Geometry: final body of the model. Coordinates: model frame, mm. A direction names the side the tool comes from. Give positions to 0.01 mm unless a question says otherwise; leave off trailing zeros. Loops run counter-clockwise (first coordinate to the right, second up) from the corner with the lowest first, then second, coordinate; pieces in that order, holes last. Notation, with made-up numbers: (50.25, -8.75) -> (92.25, -8.75) arc R16 cw to (92.25, -2.75) -> close; hole circle Ø11 at (39.25, 17.5). An arc over 180 degrees is marked (long way). Answer in a Markdown table with one row per item. Add a question column.
1) Section query B-B (y = -1.25). Return the cut outline in (x, z).
2) First-contact query: P1, Ø23.5, axis at x = 0, z = 0, coming from the +Y side; P2, Ø4, axis at y = 2.5, z = -5.5, coming from the -X side. Flat tips, straight axial feed; report the tip coordinate or a pass-through.
3) Draft query along Z for faces 3 (the flat face through (1, -3, 10)), 4 (the cylindrical face through (11.848, 2.465, -1.556)), 5 (the flat face through (0, -2.6, 2)), 6 (the cylindrical face through (2.703, 2.465, 8.584)). Return one class per face: +Z half, -Z half, draft (parallel to the pull), parting line (faces both ways), or undercut.
4) Section query A-A (y = 3.5). Return the cut outline in (x, z), plus the area to 3 significant figures.
5) Access query for faces 1 (the flat face through (9, 5, 2)), 2 (the flat face through (0, 0, 0)). Directions: +Z, -Z, +X, -X, +Y, -Y. A direction counts if a zero-diameter tool reaches every point of the face in a straight line with its end or side. Return the directions, or none.
6) Line query: line 1 (X direction, y = 2.5, z = 0); line 2 (Y direction, x = 11, z = 16.5); line 3 (Y direction, x = -6, z = 38). Output: solid intervals per line, ascending. Write a range as from..to.
```python
from build123d import *

# Parameters (mm, degrees)
SKETCH_1_R          = 11.95
SKETCH_1_R_2        = 9
EXTRUDE_1_DEPTH     = 5
SKETCH_2_R          = 44
EXTRUDE_2_DEPTH     = 3
FILLET_1_R          = 3
CUT_EXTRUDE_1_DEPTH = 0.4


with BuildPart() as part:
    # Эскиз1 → Бобышка-Вытянуть1 (new body)
    with BuildSketch(Plane(origin=(0, 0, 0), x_dir=(1, 0, 0), z_dir=(0, 1, 0))):
        with Locations(Location((0, 0, 0), (0, 0, 270))):
            Circle(SKETCH_1_R)
        with Locations(Location((0, 0, 0), (0, 0, 270))):
            Circle(SKETCH_1_R_2, mode=Mode.SUBTRACT)
    extrude(amount=EXTRUDE_1_DEPTH)

    # Эскиз2 → Бобышка-Вытянуть2 (add)
    with BuildSketch(Plane.XZ):
        with Locations(Location((0, 0, 0), (0, 0, 270))):
            Circle(SKETCH_2_R)
    extrude(amount=EXTRUDE_2_DEPTH)

    # Скругление1
    fillet_1_edges = [part.edges().sort_by_distance(p)[0] for p in [
        (0, -3, 44),
    ]]
    fillet(fillet_1_edges, radius=FILLET_1_R - 0.0001)  # a hair under: the kernel refuses the full size

    # Эскиз3 → Вырез-Вытянуть1 (cut)
    with BuildSketch(Plane.XZ.offset(3)):
        with BuildLine():
            Line((9.954559223, -5.855217729), (17.0939823, -6.624448498))
            add(Edge.make_bspline(
                [(17.0939823, -6.624448498), (16.954374573, -7.060364037), (16.67246957, -7.940593052), (16.082570182, -9.220685029), (15.367854468, -10.479237732), (14.549468275, -11.738227045), (13.598128393, -12.976714181), (12.508174471, -14.188327514), (11.307260102, -15.391109491), (9.994571436, -16.559013497), (8.599176625, -17.665541174), (7.097641414, -18.617186253), (5.53477836, -19.420340753), (3.908983058, -20.092788159), (2.213013482, -20.604345047), (0.449135236, -20.981542054), (-1.382110347, -21.198678471), (-2.625007466, -21.22599593), (-3.254575393, -21.239833113)],
                knots=[0, 0, 0, 0, 0.821440156, 1.658705401, 2.525323128, 3.419405186, 4.353419828, 5.32681938, 6.344399772, 7.404443113, 8.481060479, 9.538977106, 10.591299887, 11.633537695, 12.694215778, 13.768160887, 14.869500701, 16, 16, 16, 16], degree=3))
            add(Edge.make_bspline(
                [(-3.254575393, -21.239833113), (-4.037474252, -21.210468003), (-5.585963904, -21.152386976), (-7.859698842, -20.739484748), (-10.031214503, -20.033002378), (-12.082905697, -19.06267493), (-13.983263507, -17.838479622), (-15.628310659, -16.302835445), (-17.068788245, -14.551786811), (-18.226388665, -12.538555624), (-19.140015512, -10.335429034), (-19.780294703, -7.963227163), (-20.191471581, -5.448805692), (-20.238000287, -3.721455618), (-20.261786931, -2.838390806)],
                knots=[0, 0, 0, 0, 0.998551589, 1.975027533, 2.936744805, 3.903838964, 4.863557655, 5.807675034, 6.763178998, 7.745855275, 8.758641806, 9.797744155, 10.874151411, 12, 12, 12, 12], degree=3))
            add(Edge.make_bspline(
                [(-20.261786931, -2.838390806), (-20.253583862, -2.249072754), (-20.237148757, -1.068355571), (-20.071493014, 0.692734171), (-19.824593654, 2.443807008), (-19.457520681, 4.175543157), (-19.00443369, 5.89924412), (-18.436371871, 7.60283942), (-17.771918435, 9.296625216), (-17.009212067, 10.961487215), (-16.169576767, 12.570831605), (-15.246119859, 14.076076683), (-14.290825473, 15.491991281), (-13.257769645, 16.789715189), (-12.155533796, 17.973523587), (-11.00356969, 19.054320976), (-9.797035153, 20.040082521), (-8.518689542, 20.899962793), (-7.204489818, 21.664382583), (-5.862524589, 22.334760878), (-4.485868659, 22.886891815), (-3.083314583, 23.339978114), (-1.660006861, 23.708336607), (-0.208394214, 23.955377865), (1.268817222, 24.120842874), (2.265803014, 24.136773037), (2.767059223, 24.144782271)],
                knots=[0, 0, 0, 0, 1.075906032, 2.155611451, 3.227554832, 4.30373447, 5.38628686, 6.480642286, 7.581143633, 8.707391042, 9.82337293, 10.893692135, 11.930684225, 12.940768785, 13.919223559, 14.881988069, 15.823529777, 16.761054785, 17.692163021, 18.598508727, 19.497917784, 20.397951545, 21.288749041, 22.180057169, 23.084984307, 24, 24, 24, 24], degree=3))
            add(Edge.make_bspline(
                [(2.767059223, 24.144782271), (3.396819449, 24.13271298), (4.624674455, 24.109181262), (6.419415658, 23.873617188), (8.114533072, 23.493780483), (9.71479097, 22.957293415), (11.228369978, 22.293366902), (12.626669407, 21.438368521), (13.932702912, 20.448929523), (15.134462193, 19.318054618), (16.221199996, 18.057248477), (17.152473609, 16.665333162), (17.973572218, 15.181251724), (18.615932964, 13.571276078), (19.12246379, 11.857059969), (19.479861685, 10.030309351), (19.69885311, 8.096457894), (19.72490677, 6.769573083), (19.738213069, 6.091897656)],
                knots=[0, 0, 0, 0, 1.079196217, 2.10412856, 3.097265039, 4.052997914, 4.993829394, 5.924450447, 6.855882321, 7.798592485, 8.748507102, 9.702980304, 10.665060364, 11.651045023, 12.668191174, 13.725659051, 14.838433479, 16, 16, 16, 16], degree=3))
            add(Edge.make_bspline(
                [(19.738213069, 6.091897656), (19.711530906, 5.012347464), (19.657182115, 2.813415932), (19.336536232, 0.637210246), (19.173309223, -0.470602344)],
                knots=[0, 0, 0, 0, 0.981886135, 2, 2, 2, 2], degree=3))
            Line((19.173309223, -0.470602344), (-12.569479239, -0.470602344))
            add(Edge.make_bspline(
                [(-12.569479239, -0.470602344), (-12.686010265, -0.684825825), (-12.905708031, -1.088704703), (-13.155238164, -1.702843602), (-13.305966259, -2.286193686), (-13.328203982, -2.669377879), (-13.338710008, -2.850410037)],
                knots=[0, 0, 0, 0, 1.156942796, 2.181202349, 3.140724307, 4, 4, 4, 4], degree=3))
            add(Edge.make_bspline(
                [(-13.338710008, -2.850410037), (-13.329201362, -3.363533664), (-13.310745354, -4.359491854), (-13.176596758, -5.804983514), (-12.964076928, -7.159922166), (-12.658814238, -8.421765438), (-12.240072534, -9.58253052), (-11.763714111, -10.662876848), (-11.191471954, -11.653246376), (-10.509245809, -12.527103519), (-9.781157621, -13.313071224), (-8.993901514, -13.981427574), (-8.186858669, -14.571826363), (-7.326503521, -15.044385035), (-6.422970918, -15.399496847), (-5.487224957, -15.67198157), (-4.510031445, -15.830569123), (-3.844080664, -15.846933933), (-3.506979239, -15.855217729)],
                knots=[0, 0, 0, 0, 1.346284225, 2.613098929, 3.805631801, 4.942804233, 6.013450698, 7.039235158, 8.038108926, 9.00533571, 9.942442562, 10.84439418, 11.710848438, 12.56244313, 13.41163356, 14.253504373, 15.115931414, 16, 16, 16, 16], degree=3))
            add(Edge.make_bspline(
                [(-3.506979239, -15.855217729), (-2.858509214, -15.827358464), (-1.550821401, -15.771178193), (0.380315515, -15.234581986), (2.305705802, -14.442665665), (3.842751413, -13.498748209), (5.053499235, -12.625146746), (5.900225032, -11.858088786), (6.717542295, -11.040465602), (7.465873942, -10.135485129), (8.183042091, -9.175321866), (8.828146274, -8.133230752), (9.436128603, -7.030114624), (9.780061437, -6.250674515), (9.954559223, -5.855217729)],
                knots=[0, 0, 0, 0, 1.313044299, 2.647851039, 4.03980324, 5.527339259, 6.29475363, 7.066375866, 7.842396062, 8.63863277, 9.446691243, 10.272184996, 11.123375662, 12, 12, 12, 12], degree=3))
        make_face()
        with BuildLine():
            Line((-11.391594623, 4.91401304), (12.779078454, 4.91401304))
            add(Edge.make_bspline(
                [(12.779078454, 4.91401304), (12.787709895, 5.258551796), (12.802161832, 5.835425615), (12.811411041, 6.41240478), (12.815136146, 6.644782271)],
                knots=[0, 0, 0, 0, 1.194503009, 2, 2, 2, 2], degree=3))
            add(Edge.make_bspline(
                [(12.815136146, 6.644782271), (12.803898897, 7.117699119), (12.781959502, 8.041013127), (12.670145666, 9.384414471), (12.449186915, 10.640968329), (12.156588483, 11.815328923), (11.751690213, 12.896198212), (11.293094857, 13.905101329), (10.71543559, 14.812813231), (10.071782115, 15.638694593), (9.359494816, 16.377148538), (8.592848863, 17.01350722), (7.772383486, 17.549245443), (6.910455487, 17.999648964), (5.985412837, 18.329941166), (5.022728372, 18.590023931), (4.005305708, 18.732775986), (3.312338023, 18.750923328), (2.959366915, 18.760166887)],
                knots=[0, 0, 0, 0, 1.288915635, 2.516454775, 3.668675548, 4.762204166, 5.808675246, 6.809806692, 7.776046417, 8.732555008, 9.659000055, 10.566141369, 11.441184925, 12.324901883, 13.209090714, 14.112018255, 15.038334656, 16, 16, 16, 16], degree=3))
            add(Edge.make_bspline(
                [(2.959366915, 18.760166887), (2.569950261, 18.753640128), (1.799322271, 18.740724135), (0.659341059, 18.554273421), (-0.460843427, 18.303647562), (-1.545658439, 17.905847871), (-2.609502644, 17.425759439), (-3.649545731, 16.838318089), (-4.643906234, 16.113950662), (-5.632504092, 15.317947338), (-6.575317711, 14.401029882), (-7.44471318, 13.362562561), (-8.275005659, 12.230615841), (-9.006135858, 10.970703852), (-9.718002889, 9.624439846), (-10.328585973, 8.148804352), (-10.917153248, 6.578634088), (-11.231013188, 5.477427724), (-11.391594623, 4.91401304)],
                knots=[0, 0, 0, 0, 0.867869597, 1.717452491, 2.571772394, 3.425671253, 4.289803496, 5.174634535, 6.084973587, 7.031591473, 8.005136717, 9.013559597, 10.050697067, 11.133079613, 12.260592687, 13.446148552, 14.693362615, 16, 16, 16, 16], degree=3))
        make_face(mode=Mode.SUBTRACT)
    extrude(amount=-CUT_EXTRUDE_1_DEPTH, mode=Mode.SUBTRACT)


solid = part.part
```
Evaluation:
| question | item | result |
|---|---|---|
| 1 | outline | circle Ø87.45 at (0, 0) |
| 2 | P1 | y = 5 |
| 2 | P2 | x = -11.43 |
| 3 | face 3 | draft |
| 3 | face 4 | parting line |
| 3 | face 5 | undercut |
| 3 | face 6 | undercut |
| 4 | outline | circle Ø23.9 at (0, 0); hole circle Ø18 at (0, 0) |
| 4 | area | 194 mm² |
| 5 | face 1 | +Z, -Z, +X, -X, +Y |
| 5 | face 2 | +Y |
| 6 | line 1 | -11.95..-9, 9..11.95 |
| 6 | line 2 | -2.6..0 |
| 6 | line 3 | -3..0 |
